from build123d import *

# Parameters (mm, degrees)
SKETCH1_W               = 47.2
SKETCH1_H               = 29
SKETCH1_W_2             = 44.2
SKETCH1_H_2             = 26
BOSS_EXTRUDE2_DEPTH     = 14
SKETCH2_W               = 44.2
SKETCH2_H               = 26
BOSS_EXTRUDE3_DEPTH     = 1.5
SKETCH3_W               = 23.9
SKETCH3_H               = 7.9
SKETCH3_R               = 2.45
BOSS_EXTRUDE4_DEPTH     = 29
SKETCH4_R               = 2.5
CUT_EXTRUDE1_DEPTH      = 29
SKETCH5_R               = 3.25
CUT_EXTRUDE2_DEPTH      = 1
CUT_EXTRUDE3_START      = -1
SKETCH6_R               = 3.25
CUT_EXTRUDE3_DEPTH      = 1
CUT_EXTRUDE4_DEPTH      = 7.5
CUT_EXTRUDE4_DEPTH_BACK = 7.5
SKETCH8_R               = 3.25
SKETCH9_W               = 44.2
SKETCH9_H               = 25.968378764
SKETCH9_W_2             = 41.2
SKETCH9_H_2             = 22.968378764
BOSS_EXTRUDE5_DEPTH     = 2.5
SKETCH10_W              = 15.5
SKETCH10_H              = 1.5
SKETCH10_W_2            = 1.5
SKETCH10_H_2            = 15.5
CUT_EXTRUDE6_DEPTH      = 2
FILLET1_R               = 2
BOSS_EXTRUDE6_DEPTH     = 1.8
CUT_EXTRUDE7_REACH      = 44.52
FILLET2_R               = 0.5
FILLET3_R               = 3.6
FILLET4_R               = 1
FILLET5_R               = 3


with BuildPart() as part:
    # Sketch1 → Boss-Extrude2 (new body)
    with BuildSketch(Plane.XY):
        Rectangle(SKETCH1_W, SKETCH1_H)
        Rectangle(SKETCH1_W_2, SKETCH1_H_2, mode=Mode.SUBTRACT)
    extrude(amount=BOSS_EXTRUDE2_DEPTH)

    # Sketch2 → Boss-Extrude3 (add)
    with BuildSketch(Plane(origin=(0, 0, 0), x_dir=(-1, 0, 0), z_dir=(0, 0, -1))):
        Rectangle(SKETCH2_W, SKETCH2_H)
    extrude(amount=-BOSS_EXTRUDE3_DEPTH)

    # Sketch3 → Boss-Extrude4 (add)
    with BuildSketch(Plane.XZ.offset(14.5)):
        with Locations((0, 3.95)):
            Rectangle(SKETCH3_W, SKETCH3_H)
        with Locations(Location((-8, 3.95, 0), (0, 0, 90))):
            Circle(SKETCH3_R, mode=Mode.SUBTRACT)
        with Locations(Location((8, 3.95, 0), (0, 0, 90))):
            Circle(SKETCH3_R, mode=Mode.SUBTRACT)
    extrude(amount=-BOSS_EXTRUDE4_DEPTH)

    # Sketch4 → Cut-Extrude1 (cut)
    with BuildSketch(Plane.XZ.offset(14.5)):
        with Locations(Location((-8, 3.95, 0), (0, 0, 270))):
            Circle(SKETCH4_R)
        with Locations(Location((8, 3.95, 0), (0, 0, 270))):
            Circle(SKETCH4_R)
    extrude(amount=-CUT_EXTRUDE1_DEPTH, mode=Mode.SUBTRACT)

    # Sketch5 → Cut-Extrude2 (cut)
    with BuildSketch(Plane.XZ.offset(14.5)):
        with Locations(Location((-8, 3.95, 0), (0, 0, 270))):
            Circle(SKETCH5_R)
        with Locations(Location((8, 3.95, 0), (0, 0, 270))):
            Circle(SKETCH5_R)
    extrude(amount=-CUT_EXTRUDE2_DEPTH, mode=Mode.SUBTRACT)

    # Sketch6 → Cut-Extrude3 (cut)
    with BuildSketch(Plane(origin=(0, 14.5, 0), x_dir=(1, 0, 0), z_dir=(0, 1, 0)).offset(CUT_EXTRUDE3_START)):
        with Locations(Location((-8, -3.95, 0), (0, 0, 90))):
            Circle(SKETCH6_R)
        with Locations(Location((8, -3.95, 0), (0, 0, 90))):
            Circle(SKETCH6_R)
    extrude(amount=CUT_EXTRUDE3_DEPTH, mode=Mode.SUBTRACT)

    # Sketch8 → Cut-Extrude4 (cut, two sides: drawn at the far end of the back side and taken through both)
    with BuildSketch(Plane(origin=(0, 0, 0), x_dir=(1, 0, 0), z_dir=(0, 1, 0)).offset(-CUT_EXTRUDE4_DEPTH_BACK)):
        with Locations(Location((-8, -3.95, 0), (0, 0, 90))):
            Circle(SKETCH8_R)
        with Locations(Location((8, -3.95, 0), (0, 0, 90))):
            Circle(SKETCH8_R)
    extrude(amount=CUT_EXTRUDE4_DEPTH + CUT_EXTRUDE4_DEPTH_BACK, mode=Mode.SUBTRACT)

    # Sketch9 → Boss-Extrude5 (add)
    with BuildSketch(Plane.XY.offset(7.9)):
        Rectangle(SKETCH9_W, SKETCH9_H)
        Rectangle(SKETCH9_W_2, SKETCH9_H_2, mode=Mode.SUBTRACT)
    extrude(amount=BOSS_EXTRUDE5_DEPTH)

    # Sketch10 → Cut-Extrude6 (cut)
    with BuildSketch(Plane.XY.offset(14)):
        with Locations((0, 13.75)):
            Rectangle(SKETCH10_W, SKETCH10_H)
        with Locations((22.85, 0)):
            Rectangle(SKETCH10_W_2, SKETCH10_H_2)
        with Locations((0, -13.75)):
            Rectangle(SKETCH10_W, SKETCH10_H)
        with Locations((-22.85, 0)):
            Rectangle(SKETCH10_W_2, SKETCH10_H_2)
    extrude(amount=-CUT_EXTRUDE6_DEPTH, mode=Mode.SUBTRACT)

    # Fillet1
    fillet1_edges = [part.edges().sort_by_distance(p)[0] for p in [
        (11.95, 0, 7.9),
        (-11.95, 0, 7.9),
    ]]
    fillet(fillet1_edges, radius=FILLET1_R)

    # Sketch12 → Boss-Extrude6 (add)
    with BuildSketch(Plane.XY.offset(14)):
        Polygon((-10.839591229, 12), (-10.839591229, 13), (-12.339591229, 13), (-13.839591229, 13), (-13.839591229, 12), align=None)
        Polygon((-10.839591229, -13), (-10.839591229, -12), (-13.839591229, -12), (-13.839591229, -13), (-12.339591229, -13), align=None)
        Polygon((10.839591229, -12), (10.839591229, -13), (12.339591229, -13), (13.839591229, -13), (13.839591229, -12), align=None)
        Polygon((10.839591229, 13), (10.839591229, 12), (13.839591229, 12), (13.839591229, 13), (12.339591229, 13), align=None)
    extrude(amount=-BOSS_EXTRUDE6_DEPTH)

    # Cut-Extrude7: up to this face of the body (flat: up to its plane)
    cut_extrude7_end = Plane(part.part.faces().sort_by_distance((13.839591229, -12.5, 13.1))[0])
    # Sketch13 → Cut-Extrude7 (cut, up to the picked face)
    with BuildSketch(Plane.ZY.offset(13.839591229), mode=Mode.PRIVATE) as cut_extrude7_sk1:
        Polygon((14, 13), (14, 12), (13, 12), align=None)
    cut_extrude7_tool1 = split(extrude(cut_extrude7_sk1.sketch, amount=-CUT_EXTRUDE7_REACH, mode=Mode.PRIVATE), bisect_by=cut_extrude7_end, keep=Keep.BOTH, mode=Mode.PRIVATE)
    # Sketch13 → Cut-Extrude7 (cut, up to the picked face)
    with BuildSketch(Plane.ZY.offset(13.839591229), mode=Mode.PRIVATE) as cut_extrude7_sk2:
        Polygon((14, -13), (14, -12), (13, -12), align=None)
    cut_extrude7_tool2 = split(extrude(cut_extrude7_sk2.sketch, amount=-CUT_EXTRUDE7_REACH, mode=Mode.PRIVATE), bisect_by=cut_extrude7_end, keep=Keep.BOTH, mode=Mode.PRIVATE)
    add(cut_extrude7_tool1.solids().sort_by(Axis((-13.839591, 12.333333, 13.666667), (1, 0, 0)))[0], mode=Mode.SUBTRACT)
    add(cut_extrude7_tool2.solids().sort_by(Axis((-13.839591, -12.333333, 13.666667), (1, 0, 0)))[0], mode=Mode.SUBTRACT)

    # Fillet2
    fillet2_edges = [part.edges().sort_by_distance(p)[0] for p in [
        (-13.839591229, 13, 13.1),
        (-10.839591229, 13, 13.1),
        (10.839591229, 13, 13.1),
        (13.839591229, 13, 13.1),
        (13.839591229, -13, 13.1),
        (10.839591229, -13, 13.1),
        (-10.839591229, -13, 13.1),
        (-13.839591229, -13, 13.1),
    ]]
    fillet(fillet2_edges, radius=FILLET2_R)

    # Fillet3
    fillet3_edges = [part.edges().sort_by_distance(p)[0] for p in [
        (20.6, -11.484189382, 9.15),
        (-20.6, -11.484189382, 9.15),
        (-20.6, 11.484189382, 9.15),
        (20.6, 11.484189382, 9.15),
        (-23.6, 14.5, 7),
        (23.6, 14.5, 7),
        (23.6, -14.5, 7),
        (-23.6, -14.5, 7),
    ]]
    fillet(fillet3_edges, radius=FILLET3_R)

    # Fillet4
    fillet4_edges = [part.edges().sort_by_distance(p)[0] for p in [
        (-22.85, 7.75, 14),
        (-22.85, -7.75, 14),
        (-7.75, 13.75, 14),
        (7.75, 13.75, 14),
        (22.85, 7.75, 14),
        (22.85, -7.75, 14),
        (-7.75, -13.75, 14),
        (7.75, -13.75, 14),
    ]]
    fillet(fillet4_edges, radius=FILLET4_R)

    # Fillet5
    # the kernel refuses this fillet: 3 mm, written as the material it adds along each edge
    with BuildSketch(Plane(origin=(22.1, 13, 1.5), x_dir=(0, -1, 0), z_dir=(0, 0, 1)), Plane(origin=(22.1, -13, 1.5), x_dir=(-1, 0, 0), z_dir=(0, 0, 1))) as fillet5_piece_1:
        with BuildLine():
            CenterArc((FILLET5_R, -FILLET5_R), FILLET5_R, 90, 90)
            Line((0, -FILLET5_R), (0, 0))
            Line((0, 0), (FILLET5_R, 0))
        make_face()
    extrude(amount=12.5)
    with BuildSketch(Plane(origin=(-22.1, 13, 1.5), x_dir=(0, -1, 0), z_dir=(0, 0, 1)), Plane(origin=(-22.1, -13, 1.5), x_dir=(1, 0, 0), z_dir=(0, 0, 1))) as fillet5_piece_2:
        with BuildLine():
            CenterArc((FILLET5_R, FILLET5_R), FILLET5_R, 180, 90)
            Line((0, FILLET5_R), (0, 0))
            Line((0, 0), (FILLET5_R, 0))
        make_face()
    extrude(amount=12.5)


solid = part.part
Work out the finished part from the listing and answer in its coordinate system (mm). A direction names the side the tool comes from. Round coordinates to 2 decimals unless told otherwise and drop trailing zeros. Write each loop counter-clockwise with the first axis right and the second up, starting at its lowest first coordinate (ties: lowest second). Pieces come first, ordered by that corner, then holes. Notation, with made-up numbers: (26.25, 48.5) - (40.25, 48.5) arc R13 cw to (40.25, 54.5) - close; hole circle Ø11 at (58.25, 62). An arc over 180 degrees is marked (long way). Answer in a Markdown table with one row per item. Add a question column.
1. Given pin 1 (4 mm diameter, centred on x = 14, y = 1, fed in from +Z); pin 2 (4.5 mm diameter, centred on x = 8, z = 3.95, fed in from +Y); pin 3 (5 mm diameter, centred on x = 8, z = 4, fed in from -Y); pin 4 (2 mm diameter, centred on x = 2.5, y = -6, fed in from +Z), each flat-ended and moving along its own axis, determine where each tip first touches the part or whether it passes through.
2. Find the intervals of material crossed by line 1 along X through (y, z) = (0.75, 4); line 2 along X through (y, z) = (-2, 10.25); line 3 along Z through (x, y) = (20, -11.5), in increasing order. Write a range as from..to.
3. For faces 1 (the flat face through (7.75, 13.7, 12.5)), 2 (the flat face through (12.3, -12.5, 13.5)), 3 (the cylindrical face through (-10.44, -10.54, 4.49)), 4 (the flat face through (21, 0, 7.9)), determine the directions among +Z, -Z, +X, -X, +Y, -Y from which every point of the face is accessible in a straight line to the end or side of a thin tool.
4. A cutting plane is placed at A-A, the plane y = -4.5. Determine the outline of the cut face in (x, z), and give its area (3 significant figures).
5. The mould has two halves that part along X. Classify faces 5 (the cylindrical face through (8.051, 13.76, 13.715)), 6 (the cylindrical face through (-22.84, -8.051, 13.715)), 7 (the flat face through (23.6, 0, 7)): +X half, -X half, draft (parallel to the pull), parting line (faces both ways), or undercut.
6. A cutting plane is placed at B-B, the plane z = 3.95. Count the separate pieces of the cut face and the enclosed holes in it, and give its area (3 significant figures).
Worked out:
| question | item | result |
|---|---|---|
| 1 | pin 1 | z = 1.5 |
| 1 | pin 2 | through |
| 1 | pin 3 | y = -13.5 |
| 1 | pin 4 | z = 7.9 |
| 2 | line 1 | -23.6..-22.1, -11.95..-11.25, -4.75..4.75, 11.25..11.95, 22.1..23.6 |
| 2 | line 2 | -23.6..-20.6, 20.6..23.6 |
| 2 | line 3 | 0..1.5, 7.9..10.4 |
| 3 | face 1 | +Z, +Y, -Y |
| 3 | face 2 | +Z |
| 3 | face 3 | +Y, -Y |
| 3 | face 4 | none |
| 4 | outline | (-23.6, 0) - (23.6, 0) - (23.6, 12) - (22.1, 12) - (22.1, 10.4) - (20.6, 10.4) - (20.6, 7.9) - (22.1, 7.9) - (22.1, 1.5) - (11.95, 1.5) - (11.95, 5.9) arc R2 ccw to (9.95, 7.9) - (-9.95, 7.9) arc R2 ccw to (-11.95, 5.9) - (-11.95, 1.5) - (-22.1, 1.5) - (-22.1, 7.9) - (-20.6, 7.9) - (-20.6, 10.4) - (-22.1, 10.4) - (-22.1, 12) - (-23.6, 12) - close; hole circle Ø6.5 at (-8, 3.95); hole circle Ø6.5 at (8, 3.95) |
| 4 | area | 195 mm^2 |
| 5 | face 5 | undercut |
| 5 | face 6 | draft |
| 5 | face 7 | +X half |
| 6 | separate pieces | 3 |
| 6 | enclosed holes | 2 |
| 6 | area | 497 mm^2 |
